Check sheet for the modelled part. Datum: model origin and axes. Units: mm. Face numbers are marked on the shaded views. A direction names the side the tool comes from. Give positions to 0.01 mm unless a question says otherwise; leave off trailing zeros. Order: outer loops, then holes, each group sorted by start corner. A loop starts at its lowest first (then second) coordinate and runs counter-clockwise, first axis right, second up. Notation, with made-up numbers: (43, 13.5) - (91, 13.5) arc R15 ccw to (91, 42.5) - close; hole circle Ø9 at (63, 63). An arc over 180 degrees is marked (long way). Answer in a Markdown table with one row per item.
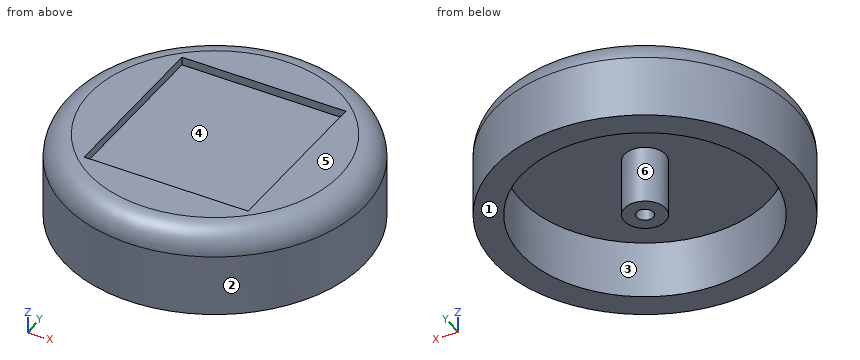
Solid Edge part; units mm, degrees
sketch "Sketch1" plane through (0, 0, 0) normal (0, 0, 1) x (1, 0, 0)
  circle A0 centre (0, 0) radius 36.5
extrude "Protrusion1" add sketch "Sketch1" along normal blind 10
sketch "Sketch2" plane through (0, 0, 0) normal (0, 0, -1) x (1, 0, 0)
  circle A0 centre (0, 0) radius 2
extrude "Extrusionsausschnitt_1" cut sketch "Sketch2" against normal blind 5
sketch "Sketch3" plane through (0, 0, 10) normal (0, 0, 1) x (0, 1, 0)
  line L0 (-21, -20) -> (21, -20)
  line L1 (21, -20) -> (21, 20)
  line L2 (21, 20) -> (-21, 20)
  line L3 (-21, 20) -> (-21, -20)
  dimension "D1" = 21
  dimension "D2" = 21
extrude "Extrusionsausschnitt_2" cut sketch "Sketch3" against normal blind 2
sketch "Sketch4" plane through (0, 0, 0) normal (0, 0, -1) x (1, 0, 0)
  circle A0 centre (0, 0) radius 2
  circle A1 centre (0, 0) radius 36.5
extrude "Extrusionsausprägung_2" add sketch "Sketch4" along normal blind 11
sketch "Sketch5" plane through (0, 0, -11) normal (0, 0, -1) x (1, 0, 0)
  circle A0 centre (0, 0) radius 30
  circle A1 centre (0, 0) radius 5
extrude "Extrusionsausschnitt_3" cut sketch "Sketch5" against normal blind 14
fillet "Verrundung_1" radius 6 1 edges at (-36.5, 0, 10)
properties material "Nylon, allgemein"
(1) Cross-section at C-C, the plane x = 0. Record the cut outline in (y, z), then the cut area to 3 significant figures.
Geometry says:
| item | result |
|---|---|
| outline | (-36.5, -11) - (-30, -11) - (-30, 3) - (-5, 3) - (-5, -11) - (-2, -11) - (-2, 5) - (2, 5) - (2, -11) - (5, -11) - (5, 3) - (30, 3) - (30, -11) - (36.5, -11) - (36.5, 4) arc R6 ccw to (30.5, 10) - (21, 10) - (21, 8) - (-21, 8) - (-21, 10) - (-30.5, 10) arc R6 ccw to (-36.5, 4) - close |
| area | 670 mm² |
(2) Mould release check, pull along Y, two halves, no side actions. Record for the marked faces 1, 2 and 3: pulls with the +Y half, pulls with the -Y half, needs draft (parallel to the pull), parting line crosses it, or undercut.
Geometry says:
| item | result |
|---|---|
| face 1 | needs draft |
| face 2 | parting line crosses it |
| face 3 | undercut |
(3) Access from +Z, -Z, +X, -X, +Y, -Y to the whole of each face (thin tool, end or side, straight path). Record for the marked faces 4, 5 and 6.
Geometry says:
| item | result |
|---|---|
| face 4 | +Z |
| face 5 | +Z, +X, -X, +Y, -Y |
| face 6 | -Z |
(4) Cross-section at D-D, the plane z = 6.25. Record the cut outline in (x, y).
Geometry says:
| item | result |
|---|---|
| outline | circle Ø72.12 at (0, 0) |
(5) Cross-section at B-B, the plane z = 0.25. Record the cut outline in (x, y), then the cut area to 3 significant figures.
Geometry says:
| item | result |
|---|---|
| outline | circle Ø73 at (0, 0); circle Ø10 at (0, 0); hole circle Ø60 at (0, 0); hole circle Ø4 at (0, 0) |
| area | 1,420 mm² |
(6) Cross-section at A-A, the plane y = 0. Record the cut outline in (x, z), then the cut area to 3 significant figures.
Geometry says:
| item | result |
|---|---|
| outline | (-36.5, -11) - (-30, -11) - (-30, 3) - (-5, 3) - (-5, -11) - (-2, -11) - (-2, 5) - (2, 5) - (2, -11) - (5, -11) - (5, 3) - (30, 3) - (30, -11) - (36.5, -11) - (36.5, 4) arc R6 ccw to (30.5, 10) - (20, 10) - (20, 8) - (-20, 8) - (-20, 10) - (-30.5, 10) arc R6 ccw to (-36.5, 4) - close |
| area | 674 mm² |
(7) Gauge pin test, flat ends, axial feed: P1, Ø0.6, axis at x = 7.5, z = 8.5, coming from the +Y side; P2, Ø20, axis at x = -0.5, y = 6, coming from the +Z side; P3, Ø5, axis at y = -13.5, z = -6.5, coming from the -X side. Record the tip position at first contact, or that the pin passes through.
Geometry says:
| item | result |
|---|---|
| P1 | y = 33.97 |
| P2 | z = 8 |
| P3 | x = -34.8 |
(8) Thickness scan on L1, parallel to Y at x = 0, z = -2; L2, parallel to Z at x = 7, y = -4. Record the ranges inside material, lowest first.
Geometry says:
| item | result |
|---|---|
| L1 | -36.5 to -30, -5 to -2, 2 to 5, 30 to 36.5 |
| L2 | 3 to 8 |
